Autodesk Inventor part; units mm, degrees
ref_plane "YZ Plane" through (0, 0, 0) normal (1, 0, 0) x (0, 1, 0)
ref_plane "XZ Plane" through (0, 0, 0) normal (0, 1, 0) x (-1, 0, 0)
ref_plane "XY Plane" through (0, 0, 0) normal (0, 0, 1) x (1, 0, 0)
sketch "Sketch1" plane through (0, 0, 0) normal (0, 1, 0) x (-1, 0, 0)
  circle A0 centre (0, 0) radius 4
  circle A1 centre (0, 0) radius 7
  dimension "d0" = 8
  dimension "d1" = 14
extrude "Extrusion1" add sketch "Sketch1" along normal blind 10
sketch "Sketch2" plane through (0, 10, 0) normal (0, 1, 0) x (1, 0, 0)
  circle A0 centre (0, 0) radius 7
  line L0 (0, -7) -> (20, -7)
  line L1 (0, 7) -> (20, 7)
  line L2 (20, 7) -> (20, -7)
  circle A1 centre (0, 0) radius 4
  arc A2 (0, 7) -> (0, -7) centre (0, 0) ccw
  dimension "d4" = 20
extrude "Extrusion2" add sketch "Sketch2" along normal blind 4
sketch "Sketch3" plane through (0, 10, 0) normal (0, -1, 0) x (1, 0, 0)
  line L0 (20, 7) -> (20, -7)
  line L1 (0, 7) -> (20, 7)
  line L2 (20, -7) -> (15, -7)
  line L3 (15, -7) -> (15, 7)
  line L4 (15, 7) -> (20, 7)
  line L5 (20, 7) -> (20, -7)
  point P0 (0, 0)
  dimension "d9" = 5
extrude "Extrusion3" add sketch "Sketch3" along normal blind 8
sketch "Sketch4" plane through (0, 2, 0) normal (0, -1, 0) x (1, 0, 0)
  circle A0 centre (17.5, -4.5) radius 2
  line L0 (20, -7) -> (20, 7)
  circle A1 centre (17.5, 4.5) radius 2
  line L1 (20, 7) -> (15, 7)
  line L2 (15, -7) -> (20, -7)
  point P0 (0, 0)
  dimension "d12" = 4
  dimension "d13" = 2.5
  dimension "d14" = 4
  dimension "d15" = 2.5
  dimension "d16" = 2.5
extrude "Extrusion4" cut sketch "Sketch4" against normal blind 15
properties part number "bedtiedown"
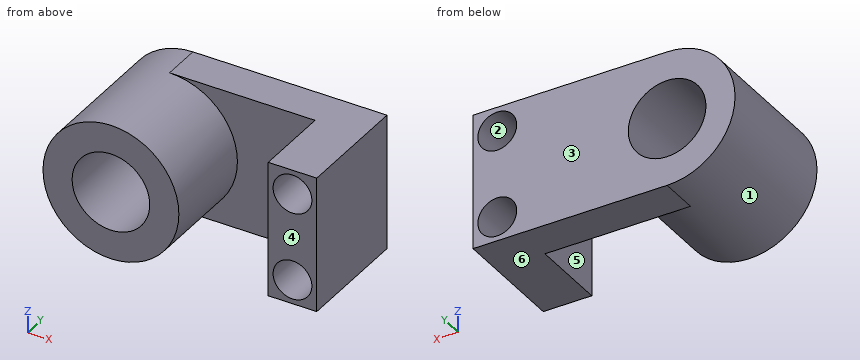
Geometry: final body of the model. Coordinates: model frame, mm. Face numbers are marked on the shaded views. A direction names the side the tool comes from. Coordinates: 2 decimals unless noted, no trailing zeros. Loops run counter-clockwise (first coordinate to the right, second up) from the corner with the lowest first, then second, coordinate; pieces in that order, holes last. Notation, with made-up numbers: M 44.25,75.25 L 52.25,75.25 A22 cw 52.25,107.25 Z; hole C 64.5,45.25 d1. An arc over 180 degrees is marked long. One line per item, written item: value. Start each with the question number.
1) Cut plane B-B (x = 17.5). Return loops of the section in (y, z), then the cut area to 3 significant figures.
2) Cut plane C-C (y = 13). Return loops of the section in (x, z).
3) Draft query along Z for the marked faces 1, 2 and 3. Return one class per face: released by +Z, released by -Z, zero draft, split by the parting line, or undercut.
4) Material intervals for L1, parallel to Z at x = 17.5, y = 7.25; L2, parallel to X at y = 5.75, z = 6.25; L3, parallel to X at y = 6.75, z = 0, sorted ascending. Write a range as from..to.
5) Cut plane D-D (z = -4.5). Return loops of the section in (x, y), then the cut area to 3 significant figures.
6) Cut plane A-A (y = 3.25). Return loops of the section in (x, z).
7) Reachability of the marked faces 4, 5 and 6 from +Z, -Z, +X, -X, +Y, -Y: full face, straight path, thin tool, end or side. Return the list, or none.
8) Pin query (flat end, axial travel): P1, Ø4.5, axis at x = 17.5, z = -4.5, coming from the +Y side; P2, Ø6.5, axis at x = 0, z = 0, coming from the -Y side; P3, Ø3, axis at x = -3.5, y = 5, coming from the +Z side; P4, Ø4, axis at x = 18, z = 1.5, coming from the -Y side. Return the tip coordinate at first contact, or that it passes through.
Evaluation:
1. outline: M 2,-7 L 14,-7 L 14,-6.5 L 2,-6.5 Z; M 2,-2.5 L 14,-2.5 L 14,2.5 L 2,2.5 Z; M 2,6.5 L 14,6.5 L 14,7 L 2,7 Z
1. area: 72.0 mm^2
2. outline: M 0,-7 L 20,-7 L 20,7 L 0,7 A7 ccw Z; hole C 0,0 d8; hole C 17.5,-4.5 d4; hole C 17.5,4.5 d4
3. face 1: split by the parting line
3. face 2: undercut
3. face 3: zero draft
4. L1: -7..-6.5, -2.5..2.5, 6.5..7
4. L2: -3.15..3.15, 15..16.53, 18.47..20
4. L3: -7..-4, 4..7, 15..20
5. outline: M -5.36,0 L 5.36,0 L 5.36,10 L 15,10 L 15,2 L 15.5,2 L 15.5,14 L -5.36,14 Z; M 19.5,2 L 20,2 L 20,14 L 19.5,14 Z
5. area: 201 mm^2
6. outline: C 0,0 d14; M 15,-7 L 20,-7 L 20,7 L 15,7 Z; hole C 0,0 d8; hole C 17.5,-4.5 d4; hole C 17.5,4.5 d4
7. face 4: +Z, -Z, +X, -Y
7. face 5: +Z, -Z, -Y
7. face 6: -Z, +X, -X, +Y, -Y
8. P1: y = 14
8. P2: through
8. P3: z = 6.71
8. P4: y = 2
